Verification items for the finished model (mm, model axes). Give positions to 0.01 mm unless a question says otherwise; leave off trailing zeros. Order: outer loops, then holes, each group sorted by start corner. A loop starts at its lowest first (then second) coordinate and runs counter-clockwise, first axis right, second up.
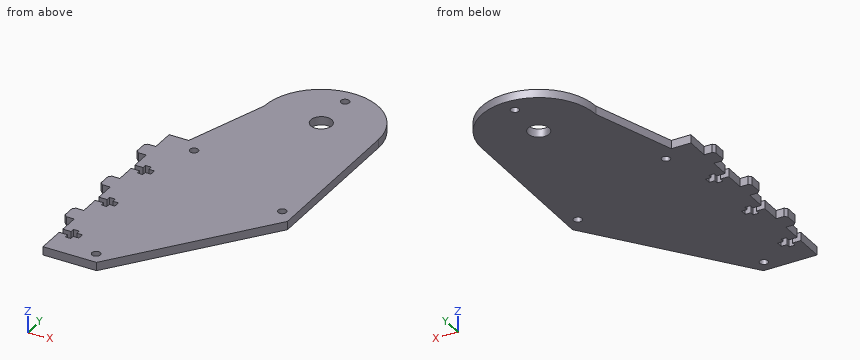
from build123d import *

# Parameters (mm, degrees)
SKETCH_1_R          = 5.03
SKETCH_1_R_2        = 2
EXTRUDE_1_DEPTH     = 4
CUT_EXTRUDE_1_DEPTH = 4


with BuildPart() as part:
    # 草图1 → 凸台-拉伸1 (new body)
    with BuildSketch(Plane.XY):
        with BuildLine():
            Line((298.551498293, -96.645689396), (302.551498293, -96.645689396))
            Line((302.551498293, -96.645689396), (302.551498293, -98.644151028))
            Line((302.551498293, -98.644151028), (305.251498293, -98.644151028))
            Line((305.251498293, -98.644151028), (305.251498293, -96.645689396))
            Line((305.251498293, -96.645689396), (307.951498293, -96.645689396))
            Line((307.951498293, -96.645689396), (307.951498293, -93.645689396))
            Line((307.951498293, -93.645689396), (305.251498293, -93.645689396))
            Line((305.251498293, -93.645689396), (305.251498293, -91.647227763))
            Line((305.251498293, -91.647227763), (302.551498293, -91.647227763))
            Line((302.551498293, -91.647227763), (302.551498293, -93.645689396))
            Line((302.551498293, -93.645689396), (298.551498293, -93.645689396))
            Line((298.551498293, -93.645689396), (298.551498293, -84.145716775))
            Line((298.551498293, -84.145716775), (293.551498293, -84.145716775))
            Line((293.551498293, -84.145716775), (293.551498293, -76.145716775))
            Line((293.551498293, -76.145716775), (298.551498293, -76.145716775))
            Line((298.551498293, -76.145716775), (298.551498293, -66.645694374))
            Line((298.551498293, -66.645694374), (302.551498293, -66.645694374))
            Line((302.551498293, -66.645694374), (302.551498293, -68.644156006))
            Line((302.551498293, -68.644156006), (305.251498293, -68.644156006))
            Line((305.251498293, -68.644156006), (305.251498293, -66.645694374))
            Line((305.251498293, -66.645694374), (307.951498293, -66.645694374))
            Line((307.951498293, -66.645694374), (307.951498293, -63.645694374))
            Line((307.951498293, -63.645694374), (305.251498293, -63.645694374))
            Line((305.251498293, -63.645694374), (305.251498293, -61.647232741))
            Line((305.251498293, -61.647232741), (302.551498293, -61.647232741))
            Line((302.551498293, -61.647232741), (302.551498293, -63.645694374))
            Line((302.551498293, -63.645694374), (298.551498293, -63.645694374))
            Line((298.551498293, -63.645694374), (298.551498293, -54.145671973))
            Line((298.551498293, -54.145671973), (293.551498293, -54.145671973))
            Line((293.551498293, -54.145671973), (293.551498293, -46.145671973))
            Line((293.551498293, -46.145671973), (298.551498293, -46.145671973))
            Line((298.551498293, -46.145671973), (298.551498293, -35.045714286))
            Line((298.551498293, -35.045714286), (307.942857143, -35.045714286))
            Line((307.942857143, -35.045714286), (321.159325739, 4.854285714))
            ThreePointArc((321.159325739, 4.854285714), (348.542857143, 32.081451417), (375.926388547, 4.854285714))
            Line((375.926388547, 4.854285714), (376.364473934, -71.645714286))
            Line((376.364473934, -71.645714286), (324.194731876, -140.145734198))
            Line((324.194731876, -140.145734198), (298.551498293, -140.145734198))
            Line((298.551498293, -140.145734198), (298.551498293, -126.645734198))
            Line((298.551498293, -126.645734198), (302.551498293, -126.645734198))
            Line((302.551498293, -126.645734198), (302.551498293, -128.644195831))
            Line((302.551498293, -128.644195831), (305.251498293, -128.644195831))
            Line((305.251498293, -128.644195831), (305.251498293, -126.645734198))
            Line((305.251498293, -126.645734198), (307.951498293, -126.645734198))
            Line((307.951498293, -126.645734198), (307.951498293, -123.645734198))
            Line((307.951498293, -123.645734198), (305.251498293, -123.645734198))
            Line((305.251498293, -123.645734198), (305.251498293, -121.647272565))
            Line((305.251498293, -121.647272565), (302.551498293, -121.647272565))
            Line((302.551498293, -121.647272565), (302.551498293, -123.645734198))
            Line((302.551498293, -123.645734198), (298.551498293, -123.645734198))
            Line((298.551498293, -123.645734198), (298.551498293, -114.145711797))
            Line((298.551498293, -114.145711797), (293.551498293, -114.145711797))
            Line((293.551498293, -114.145711797), (293.551498293, -106.145711797))
            Line((293.551498293, -106.145711797), (298.551498293, -106.145711797))
            Line((298.551498293, -106.145711797), (298.551498293, -96.645689396))
        make_face()
        with Locations((348.542857143, 4.854285714)):
            Circle(SKETCH_1_R, mode=Mode.SUBTRACT)
        with Locations((348.542857143, 24.697471009)):
            Circle(SKETCH_1_R_2, mode=Mode.SUBTRACT)
        with Locations((320.551498293, -134.145734198)):
            Circle(SKETCH_1_R_2, mode=Mode.SUBTRACT)
        with Locations((370.364473934, -65.645714286)):
            Circle(SKETCH_1_R_2, mode=Mode.SUBTRACT)
        with Locations((313.942857143, -41.045714286)):
            Circle(SKETCH_1_R_2, mode=Mode.SUBTRACT)
    extrude(amount=EXTRUDE_1_DEPTH)

    # 草图3 → 切除-拉伸1 (cut)
    with BuildSketch(Plane.XY.offset(4)):
        Polygon((293.551498293, -46.145671973), (294.751498293, -46.145671973), (293.551498293, -47.345671973), align=None)
        Polygon((294.751498293, -84.145716775), (293.551498293, -84.145716775), (293.551498293, -82.945716775), align=None)
        Polygon((293.551498293, -77.345716775), (293.551498293, -76.145716775), (294.751498293, -76.145716775), align=None)
        Polygon((294.751498293, -54.145671973), (293.551498293, -54.145671973), (293.551498293, -52.945671973), align=None)
        Polygon((293.551498293, -114.145711797), (293.551498293, -112.945711797), (294.751498293, -114.145711797), align=None)
        Polygon((293.551498293, -107.345711797), (293.551498293, -106.145711797), (294.751498293, -106.145711797), align=None)
    extrude(amount=-CUT_EXTRUDE_1_DEPTH, mode=Mode.SUBTRACT)


solid = part.part
(1) Scan lines: line 1 (Y direction, x = 300, z = 1.25); line 2 (Y direction, x = 349, z = 1.7); line 3 (Y direction, x = 346.5, z = 3.1). Record each from-to range of solid material in increasing order.
Solved:
line 1: y = -140.15 to -126.65, -123.65 to -96.65, -93.65 to -66.65, -63.65 to -35.05
line 2: y = -107.58 to -0.15, 9.86 to 22.75, 26.64 to 32.08
line 3: y = -110.86 to 0.26, 9.45 to 32.01
(2) Go/stop test with flat-tipped pins: pin 1 (2 mm diameter, centred on x = 303.5, z = 2, fed in from +Y); pin 2 (2 mm diameter, centred on y = -92.5, z = 2.5, fed in from +X); pin 3 (1 mm diameter, centred on x = 336, z = 2.5, fed in from -Y); pin 4 (3 mm diameter, centred on x = 313.94, y = -41.05, fed in from -Z). Record where each tip stops, or that it passes through.
Solved:
pin 1: stops at y = -35.05
pin 2: stops at x = 361.24
pin 3: stops at y = -125.3
pin 4: passes through
(3) Section check C-C, the plane z = 1.6. Give the number of separate pieces and of enclosed holes in the cut face, then the cut area to 3 significant figures.
Solved:
separate pieces: 1
enclosed holes: 5
area: 9,880 mm2
(4) Section check B-B, the plane x = 328. Enter the section's corners in (y, z).
Solved:
outline: (-135.15, 0) - (22.8, 0) - (22.8, 4) - (-135.15, 4) - close
(5) Section check A-A, the plane y = 19.5. Enter the section's corners in (x, z), then the cut area to 3 significant figures.
Solved:
outline: (325.5, 0) - (371.58, 0) - (371.58, 4) - (325.5, 4) - close
area: 184 mm2
